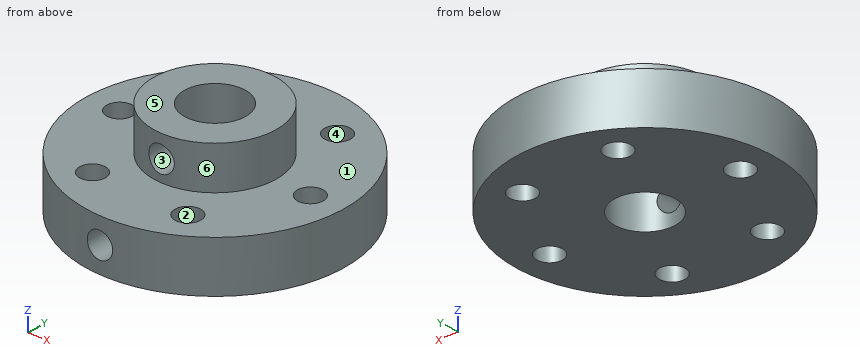
Autodesk Fusion 360 part; units mm, degrees
sketch "Esquisse1" plane through (0, 0, 0) normal (0, 0, 1) x (1, 0, 0)
  circle A0 centre (0, 0) radius 12.7
  circle A1 centre (0, 0) radius 6
  circle A2 centre (0, 0) radius 3
  dimension "d1" = 25.4
  dimension "d2" = 12
  dimension "d3" = 6
extrude "Extrusion1" add sketch "Esquisse1" along normal blind 5 contours A0
extrude "Extrusion2" add sketch "Esquisse1" along normal blind 9.2 contours A1
sketch "Esquisse2" plane through (0, 0, 5) normal (0, 0, 1) x (-1, 0, 0)
  circle A0 centre (0, 0) radius 6
  circle A1 centre (0, 0) radius 12.7
  circle A2 centre (0, 0) radius 9.5
  circle A3 centre (-9.5, 0) radius 0.445
  circle A4 centre (-4.75, -8.2272) radius 0.445
  circle A5 centre (4.75, -8.2272) radius 0.445
  circle A6 centre (9.5, 0) radius 0.445
  circle A7 centre (4.75, 8.2272) radius 0.445
  circle A8 centre (-4.75, 8.2272) radius 0.445
  point P0 (-4.75, -8.2272)
  point P1 (4.75, -8.2272)
  point P2 (9.5, 0)
  point P3 (4.75, 8.2272)
  point P4 (-4.75, 8.2272)
  dimension "d8" = 19
  dimension "d10" = 0.89
  dimension "d12" = 360
  dimension "d13" = 0.89
  dimension "d14" = 0.89
  dimension "d15" = 0.89
  dimension "d16" = 0.89
  dimension "d17" = 0.89
hole "Perçage1" at (4.75, 8.2272, 5) at (-4.75, 8.2272, 5) at (-9.5, 0, 5) at (-4.75, -8.2272, 5) at (4.75, -8.2272, 5) at (9.5, 0, 5) direction (0, 0, -1) diameter 2.529 depth 6 tip angle 118
sketch "Esquisse3" plane through (0, 0, 0) normal (0, 1, 0) x (1, 0, 0)
  circle A0 centre (0, -2.5) radius 0.445
  circle A1 centre (0, -7) radius 0.445
  dimension "d23" = 0.89
  dimension "d24" = 0.89
hole "Perçage2" at (0, 0, 7) at (0, 0, 2.5) direction (0, -1, 0) diameter 2.529 depth 22.5 tip angle 118
The model under review builds one solid part; all positions refer to its coordinate system, in mm. Face numbers are marked on the shaded views. A direction names the side the tool comes from. Give positions to 0.01 mm unless a question says otherwise; leave off trailing zeros. Write each loop counter-clockwise with the first axis right and the second up, starting at its lowest first coordinate (ties: lowest second). Pieces come first, ordered by that corner, then holes. Notation, with made-up numbers: M 86.5,14.25 L 128.5,14.25 A8 cw 128.5,22.25 Z; hole C 55,-30.75 d1. An arc over 180 degrees is marked long. Write item = value, one per line. Start each with the question number.
Q1. We need section A-A (y = 0). State the section outline as (x, z) points, plus the area to 3 significant figures.
Q2. Mouldability with a two-part tool opening along Y and no side actions: class the marked faces 4, 5 and 6 as released by +Y, released by -Y, zero draft, split by the parting line, or undercut.
Q3. Machinability: for the marked faces 1, 2 and 3, which of the approach directions +Z, -Z, +X, -X, +Y, -Y give a long, thin tool a straight path to every point of the face, cutting with its end or side? Answer none if there is none.
Q4. Clearance check with flat-ended pins moving along their axes: pin 1 (1 mm diameter, centred on x = 7, z = 1.5, fed in from -Y); pin 2 (2.5 mm diameter, centred on x = 0, z = 7, fed in from +Y); pin 3 (3 mm diameter, centred on x = 9.5, y = 0, fed in from +Z). State where each tip first meets the part, or that it passes through.
Q5. For line 1 (Z direction, x = 0, y = -10); line 2 (X direction, y = 9.25, z = 4.25); line 3 (Y direction, x = -4.5, z = 4.5), list the stretches that pass through material, from the lowest coordinate up.
Q6. We need section C-C (x = -4.75). State the section outline as (y, z) points, plus the area to 3 significant figures.
Q7. We need section B-B (x = 0). State the section outline as (y, z) points, plus the area to 3 significant figures.
Q8. We need section D-D (z = 3). State the section outline as (x, y) points.
Result set:
q1.outline = M -12.7,0 L -10.76,0 L -10.76,5 L -12.7,5 Z; M -8.24,0 L -3,0 L -3,9.2 L -6,9.2 L -6,5 L -8.24,5 Z; M 3,0 L 8.24,0 L 8.24,5 L 6,5 L 6,9.2 L 3,9.2 Z; M 10.76,0 L 12.7,0 L 12.7,5 L 10.76,5 Z
q1.area = 96.9 mm2
q2.face_4 = undercut
q2.face_5 = zero draft
q2.face_6 = split by the parting line
q3.face_1 = +Z
q3.face_2 = +Z, -Z
q3.face_3 = -Y
q4.pin_1 = -10.91
q4.pin_2 = 6
q4.pin_3 = 5
q5.line_1 = 0 to 1.24, 3.76 to 5
q5.line_2 = -8.7 to -5.49, -4.01 to 4.01, 5.49 to 8.7
q5.line_3 = -11.88 to -9.47, -6.99 to 6.99, 9.47 to 11.88
q6.outline = M -11.78,0 L -9.49,0 L -9.49,5 L -11.78,5 Z; M -6.96,0 L 6.96,0 L 6.96,5 L 3.67,5 L 3.67,9.2 L -3.67,9.2 L -3.67,5 L -6.96,5 Z; M 9.49,0 L 11.78,0 L 11.78,5 L 9.49,5 Z
q6.area = 123 mm2
q7.outline = M -12.7,0 L -3,0 L -3,1.24 L -12.7,1.24 Z; M -12.7,3.76 L -3,3.76 L -3,5.74 L -6,5.74 L -6,5 L -12.7,5 Z; M -6,8.26 L -3,8.26 L -3,9.2 L -6,9.2 Z; M 3,0 L 12.7,0 L 12.7,5 L 6,5 L 6,9.2 L 3,9.2 Z
q7.area = 90.1 mm2
q8.outline = M -1.16,-12.65 L -1.16,-2.77 A3 cw long 1.16,-2.77 L 1.16,-12.65 A12.7 ccw long Z; hole C -9.5,0 d2.53; hole C -4.75,-8.23 d2.53; hole C -4.75,8.23 d2.53; hole C 4.75,-8.23 d2.53; hole C 4.75,8.23 d2.53; hole C 9.5,0 d2.53
